Verification items for the finished model (mm, model axes). A direction names the side the tool comes from. Give positions to 0.01 mm unless a question says otherwise; leave off trailing zeros. Order: outer loops, then holes, each group sorted by start corner. A loop starts at its lowest first (then second) coordinate and runs counter-clockwise, first axis right, second up. Notation, with made-up numbers: (-38.5, -20) -> (-27.5, -20) arc R21 ccw to (-27.5, -6) -> close; hole circle Ø1 at (-36.5, 23). An arc over 180 degrees is marked (long way). One line per question, with ' | ' between items. Start each with the question number.
Q1. Section check B-B on z = 58. Record the cut outline in (x, y).
Q2. Section check D-D on z = 32. Record the cut outline in (x, y).
Q3. Section check C-C on y = 10. Record the cut outline in (x, z).
Q4. Go/stop test with flat-tipped pins: pin 1 (4 mm diameter, centred on x = 82, y = 11, fed in from +Z); pin 2 (2.5 mm diameter, centred on y = -9.5, z = 1.5, fed in from +X); pin 3 (11 mm diameter, centred on x = 0, y = -13, fed in from +Z); pin 4 (4 mm diameter, centred on x = 71.5, y = 3.5, fed in from +Z). Record where each tip stops, or that it passes through.
Q5. Access from +Z, -Z, +X, -X, +Y, -Y to the whole of each face (thin tool, end or side, straight path). Record for faces 5 (the flat face through (150, 0, 12)), 6 (the flat face through (0, 0, 0)), 7 (the flat face through (145, 0, 45)).
Q6. Material ranges on probe 1 along Y at (x, z) = (160, 66); probe 2 along Y at (x, z) = (127.5, 0); probe 3 along Z at (x, y) = (55, -3), recorded low to high. Write a range as [from, to].
Q7. Mould release check, pull along X, two halves, no side actions. Record for faces 1 (the flat face through (71, 0, 10)), 2 (the flat face through (5, -10, 0)), 3 (the cylindrical face through (-0.26, -10.517, -0.07)), 4 (the flat face through (144, 0, 27)): released by +X, released by -X, zero draft, split by the parting line, or undercut.
Q8. Section check A-A on x = 160. Record the cut outline in (y, z), plus the area to 3 significant figures.
from build123d import *

# Parameters (mm, degrees)
SKETCH4_W                = 20
SKETCH4_H                = 15
BOSS_EXTRUDE1_DEPTH      = 150
SKETCH5_W                = 6
SKETCH5_H                = 15
BOSS_EXTRUDE2_DEPTH      = 35
SKETCH6_R                = 14.5
SKETCH6_R_2              = 6.5
BOSS_EXTRUDE3_DEPTH      = 35
BOSS_EXTRUDE3_DEPTH_BACK = 10
SKETCH7_R                = 2
BOSS_EXTRUDE4_DEPTH      = 5
FILLET1_R                = 2


with BuildPart() as part:
    # Sketch4 → Boss-Extrude1 (new body)
    with BuildSketch(Plane(origin=(0, 0, 0), x_dir=(0, 0, -1), z_dir=(1, 0, 0))):
        Rectangle(SKETCH4_W, SKETCH4_H)
    extrude(amount=BOSS_EXTRUDE1_DEPTH)

    # Sketch5 → Boss-Extrude2 (add)
    with BuildSketch(Plane.XY.offset(10)):
        with Locations((147, 0)):
            Rectangle(SKETCH5_W, SKETCH5_H)
    extrude(amount=BOSS_EXTRUDE2_DEPTH)

    # Sketch6 → Boss-Extrude3 (add, two sides)
    with BuildSketch(Plane.XY.offset(45)) as boss_extrude3_sk:
        with Locations((160, 0)):
            Circle(SKETCH6_R)
        with Locations((160, 0)):
            Circle(SKETCH6_R_2, mode=Mode.SUBTRACT)
    extrude(amount=BOSS_EXTRUDE3_DEPTH)
    extrude(boss_extrude3_sk.sketch, amount=-BOSS_EXTRUDE3_DEPTH_BACK)

    # Sketch7 → Boss-Extrude4 (add, symmetric)
    with BuildSketch(Plane.XY):
        with BuildLine():
            Line((5, -12.5), (5, -7.5))
            Line((5, -7.5), (0, -7.5))
            ThreePointArc((0, -7.5), (-3.535533906, -16.035533906), (5, -12.5))
        make_face()
        with Locations((0, -12.5)):
            Circle(SKETCH7_R, mode=Mode.SUBTRACT)
    extrude(amount=BOSS_EXTRUDE4_DEPTH, both=True)

    # Fillet1
    fillet1_edges = [part.edges().sort_by_distance(p)[0] for p in [
        (0, -7.5, -7.5),
        (0, -7.5, 7.5),
    ]]
    fillet(fillet1_edges, radius=FILLET1_R)


solid = part.part
Filled in:
1) outline: circle Ø29 at (160, 0); hole circle Ø13 at (160, 0)
2) outline: (144, -7.5) -> (150, -7.5) -> (150, 7.5) -> (144, 7.5) -> close
3) outline: (149.5, 35) -> (170.5, 35) -> (170.5, 80) -> (149.5, 80) -> close
4) pin 1: through | pin 2: x = 5 | pin 3: z = 5 | pin 4: z = 10
5) face 5: -Z, +X, +Y, -Y | face 6: +Z, -Z, -X, +Y | face 7: +Z, -X
6) probe 1: [-14.5, -6.5], [6.5, 14.5] | probe 2: [-7.5, 7.5] | probe 3: [-10, 10]
7) face 1: zero draft | face 2: released by +X | face 3: undercut | face 4: released by -X
8) outline: (-14.5, 35) -> (-6.5, 35) -> (-6.5, 80) -> (-14.5, 80) -> close; (6.5, 35) -> (14.5, 35) -> (14.5, 80) -> (6.5, 80) -> close | area: 720 mm²
